Can you work these out from the model? Positions are in its coordinate system, mm. Coordinates: 2 decimals unless noted, no trailing zeros. Loops run counter-clockwise (first coordinate to the right, second up) from the corner with the lowest first, then second, coordinate; pieces in that order, holes last.
```python
from build123d import *

# Parameters (mm, degrees)
ESQUISSE1_R             = 2.5
ESQUISSE1_R_2           = 2.1
BOSS_EXTRU_1_DEPTH      = 3
ESQUISSE2_R             = 1.6
ENL_V_MAT_EXTRU_1_DEPTH = 53.28766585


with BuildPart() as part:
    # Esquisse1 → Boss.-Extru.1 (new body)
    with BuildSketch(Plane.XY):
        with BuildLine():
            Line((-35, 15), (35, 15))
            ThreePointArc((35, 15), (50, 0), (35, -15))
            Line((35, -15), (-35, -15))
            ThreePointArc((-35, -15), (-50, 0), (-35, 15))
        make_face()
        with Locations((35, 0)):
            Circle(ESQUISSE1_R, mode=Mode.SUBTRACT)
        with Locations((-35, 0)):
            Circle(ESQUISSE1_R_2, mode=Mode.SUBTRACT)
    extrude(amount=BOSS_EXTRU_1_DEPTH)

    # Esquisse2 → Enlèv. mat.-Extru.1 (cut, through all)
    with BuildSketch(Plane.XY.offset(3)):
        with Locations((35, 10)):
            Circle(ESQUISSE2_R)
        with Locations(Location((35, -10, 0), (0, 0, 180))):
            Circle(ESQUISSE2_R)
    extrude(amount=-ENL_V_MAT_EXTRU_1_DEPTH, mode=Mode.SUBTRACT)


solid = part.part
```
(1) I want a section at D-D on y = 5. Write out the boundary of the cut face in (x, z), then the cut area to 3 significant figures.
Check values:
outline: (-49.14, 0) - (49.14, 0) - (49.14, 3) - (-49.14, 3) - close
area: 295 mm2
(2) I want a section at A-A on z = 1.15. Write out the boundary of the cut face in (x, y).
Check values:
outline: (-35, -15) - (35, -15) arc R15 ccw to (35, 15) - (-35, 15) arc R15 ccw to start; hole circle Ø4.2 at (-35, 0); hole circle Ø5 at (35, 0); hole circle Ø3.2 at (35, -10); hole circle Ø3.2 at (35, 10)
(3) I want a section at C-C on y = 10. Write out the boundary of the cut face in (x, z).
Check values:
outline: (-46.18, 0) - (33.4, 0) - (33.4, 3) - (-46.18, 3) - close; (36.6, 0) - (46.18, 0) - (46.18, 3) - (36.6, 3) - close
(4) I'm going to push flat-ended pins straight in: pin 1 (10 mm diameter, centred on x = -21, y = 10, fed in from -Z); pin 2 (1.5 mm diameter, centred on y = 7, z = 2, fed in from +X); pin 3 (3 mm diameter, centred on x = 35, y = 0, fed in from -Z); pin 4 (1.5 mm diameter, centred on y = 1, z = 2, fed in from -X). Where does each tip first touch, or does it pass through?
Check values:
pin 1: stops at z = 0
pin 2: stops at x = 48.64
pin 3: passes through
pin 4: stops at x = -50
(5) I want a section at B-B on y = 0. Write out the boundary of the cut face in (x, z).
Check values:
outline: (-50, 0) - (-37.1, 0) - (-37.1, 3) - (-50, 3) - close; (-32.9, 0) - (32.5, 0) - (32.5, 3) - (-32.9, 3) - close; (37.5, 0) - (50, 0) - (50, 3) - (37.5, 3) - close
(6) If we mould it in two halves opening along Y, with no side actions, what happens to faces 1 (the cylindrical face through (-37.1, 0.09, 1.48)), 2 (the flat face through (0, 15, 1)), 3 (the cylindrical face through (50, 0, 1))? For each: released by +Y, released by -Y, zero draft, split by the parting line, or undercut.
Check values:
face 1: undercut
face 2: released by +Y
face 3: split by the parting line
(7) If I drill on probe 1 along Y at (x, z) = (35, 1.4); probe 2 along X at (y, z) = (-0.5, 0.7); probe 3 along Y at (x, z) = (34.5, 2.4), over which ranges is the centre line in solid material (lowest first)?
Check values:
probe 1: y = -15 to -11.6, -8.4 to -2.5, 2.5 to 8.4, 11.6 to 15
probe 2: x = -49.99 to -37.04, -32.96 to 32.55, 37.45 to 49.99
probe 3: y = -15 to -11.52, -8.48 to -2.45, 2.45 to 8.48, 11.52 to 15
